The drawing under review shows one solid part. Ordinate dimensions are in mm from its lowest x, y, z. Round coordinates to 2 decimals unless told otherwise and drop trailing zeros. Loops run counter-clockwise (first coordinate to the right, second up) from the corner with the lowest first, then second, coordinate; pieces in that order, holes last. Notation, with made-up numbers: M 72,84 L 92,84 A27 ccw 92,120 Z; hole C -24.75,17 d11. An arc over 180 degrees is marked long. Use a Markdown table: item, result.
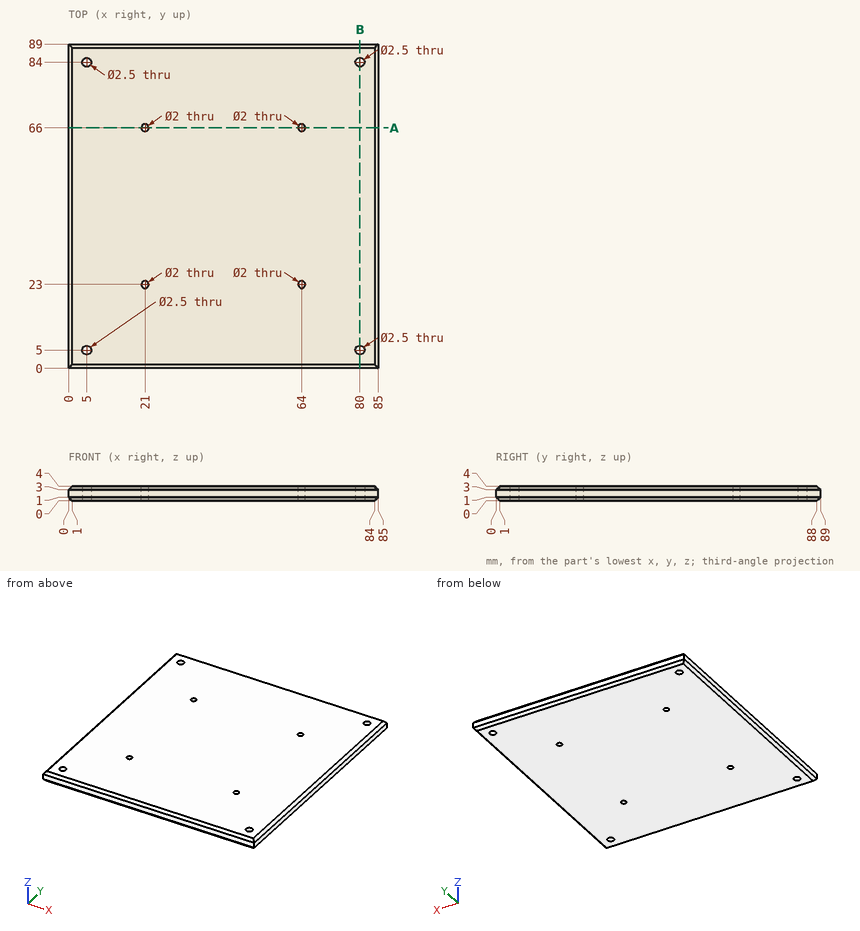
1. Insertion check: pin 1 (1.5 mm diameter, centred on x = 5, y = 5, fed in from +Z). The pin has a flat end and moves straight along its axis. Give the tip position at first contact, or say it passes through.
Check values:
| item | result |
|---|---|
| pin 1 | passes through |
2. Take a section at B-B on x = 80. Give the boundary of the cut face in (y, z), and give its area (3 significant figures).
Check values:
| item | result |
|---|---|
| outline | M 0,1 L 1,0 L 3.75,0 L 3.75,4 L 1,4 L 0,3 Z; M 6.25,0 L 82.75,0 L 82.75,4 L 6.25,4 Z; M 85.25,0 L 88,0 L 89,1 L 89,3 L 88,4 L 85.25,4 Z |
| area | 334 mm² |
3. Take a section at A-A on y = 66. Give the boundary of the cut face in (x, z).
Check values:
| item | result |
|---|---|
| outline | M 0,1 L 1,0 L 20,0 L 20,4 L 1,4 L 0,3 Z; M 22,0 L 63,0 L 63,4 L 22,4 Z; M 65,0 L 84,0 L 85,1 L 85,3 L 84,4 L 65,4 Z |
4. Wall thickness on line 1 along X through (y, z) = (5, 2.3); line 2 along Y through (x, z) = (21, 1.45); line 3 along X through (y, z) = (66, 2.55): over which ranges is each line inside the solid? List them lowest first. Write a range as from..to.
Check values:
| item | result |
|---|---|
| line 1 | x = 0..3.75, 6.25..78.75, 81.25..85 |
| line 2 | y = 0..22, 24..65, 67..89 |
| line 3 | x = 0..20, 22..63, 65..85 |
